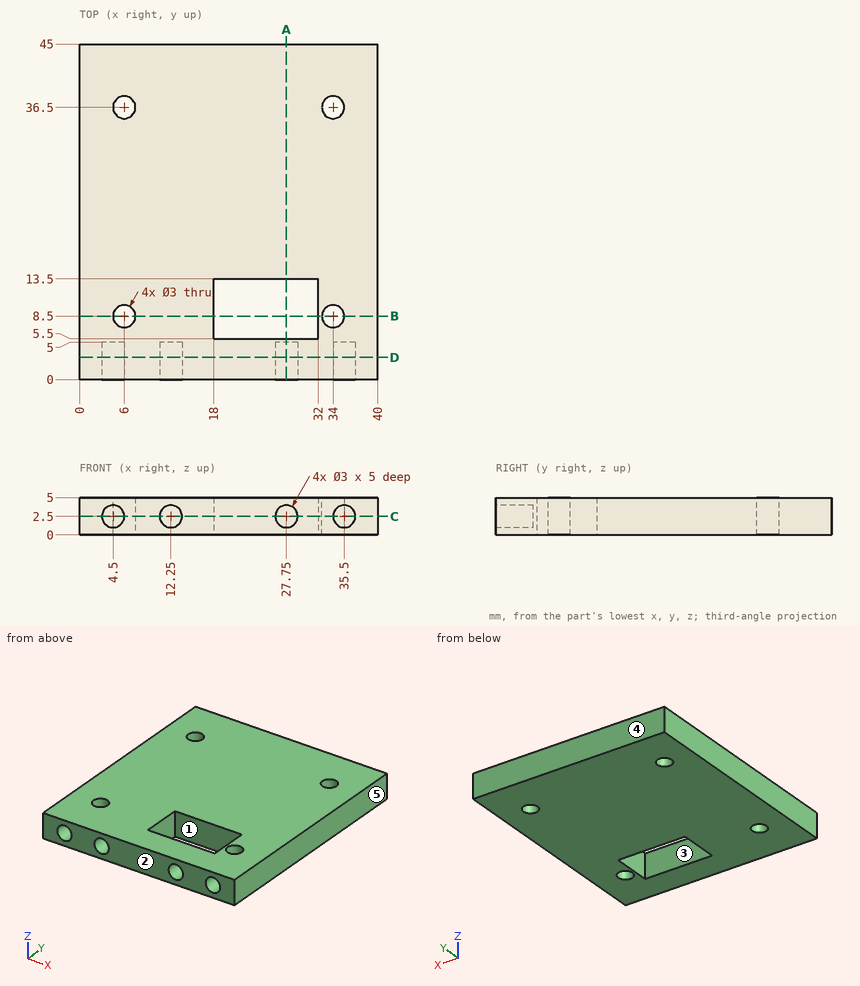
Job drawing, mm, ordinate dimensions from the low corner. One solid piece. A direction names the side the tool comes from. Give positions to 0.01 mm unless a question says otherwise; leave off trailing zeros. Loops run counter-clockwise (first coordinate to the right, second up) from the corner with the lowest first, then second, coordinate; pieces in that order, holes last. Notation, with made-up numbers: M -24,-24 L -2,-24 A36 cw -2,14 Z; hole C 56,88 d10. An arc over 180 degrees is marked long. Return JSON: item names as keys, results as strings.
1) Saw through at A-A, the plane x = 27.75. List the corners of the cut face in (y, z), then the cut area to 3 significant figures.
Calculated:
{"outline": "M 0,0 L 5.5,0 L 5.5,5 L 0,5 L 0,4 L 5,4 L 5,1 L 0,1 Z; M 13.5,0 L 45,0 L 45,5 L 13.5,5 Z", "area": "170 mm2"}
2) Saw through at D-D, the plane y = 3. List the corners of the cut face in (x, z).
Calculated:
{"outline": "M 0,0 L 40,0 L 40,5 L 0,5 Z; hole C 4.5,2.5 d3; hole C 12.25,2.5 d3; hole C 27.75,2.5 d3; hole C 35.5,2.5 d3"}
3) Flat gauge pin, fed straight in: pin 1 Ø0.9 at (x, z) = (35, 3) entering from -Y. Where does the tip first touch, or does it go through?
Calculated:
{"pin 1": "stops at y = 5"}
4) Drill centre lines: line 1 (Y direction, x = 34, z = 1.85); line 2 (X direction, y = 3.5, z = 2.5); line 3 (Y direction, x = 5.5, z = 0.8). Where is each one in solid material? Low to high.
Calculated:
{"line 1": "y = 0 to 7, 10 to 35, 38 to 45", "line 2": "x = 0 to 3, 6 to 10.75, 13.75 to 26.25, 29.25 to 34, 37 to 40", "line 3": "y = 0 to 7.09, 9.91 to 35.09, 37.91 to 45"}
5) Saw through at B-B, the plane y = 8.5. List the corners of the cut face in (x, z).
Calculated:
{"outline": "M 0,0 L 4.5,0 L 4.5,5 L 0,5 Z; M 7.5,0 L 18,0 L 18,5 L 7.5,5 Z; M 32,0 L 32.5,0 L 32.5,5 L 32,5 Z; M 35.5,0 L 40,0 L 40,5 L 35.5,5 Z"}
6) Saw through at C-C, the plane z = 2.5. List the corners of the cut face in (x, y), then the cut area to 3 significant figures.
Calculated:
{"outline": "M 0,0 L 3,0 L 3,5 L 6,5 L 6,0 L 10.75,0 L 10.75,5 L 13.75,5 L 13.75,0 L 26.25,0 L 26.25,5 L 29.25,5 L 29.25,0 L 34,0 L 34,5 L 37,5 L 37,0 L 40,0 L 40,45 L 0,45 Z; hole C 6,8.5 d3; hole C 6,36.5 d3; hole M 18,5.5 L 32,5.5 L 32,13.5 L 18,13.5 Z; hole C 34,8.5 d3; hole C 34,36.5 d3", "area": "1,600 mm2"}
7) 3-axis set-ups, long thin cutter, end or side, ignore diameter. For the marked faces 1 and 2: which of +Z, -Z, +X, -X, +Y, -Y reach the whole face in a straight line?
Calculated:
{"face 1": "+Z, -Z", "face 2": "+Z, -Z, +X, -X, -Y"}
8) Pull direction X, two halves, no side cores. Call the marked faces 3, 4 and 5: released by +X, released by -X, zero draft, split by the parting line, or undercut.
Calculated:
{"face 3": "undercut", "face 4": "zero draft", "face 5": "released by +X"}
